from build123d import *

# Parameters (mm, degrees)
F0_W     = 66.675
F0_H     = 101.6
F1_DEPTH = 0.79375


with BuildPart() as f1:
    # F0 (on Front) → F1 (new body, symmetric)
    with BuildSketch(Plane.XZ):
        with BuildLine():
            Line((117.475, 114.3), (-117.475, 114.3))
            ThreePointArc((-117.475, 114.3), (-126.455256, 110.580256), (-130.175, 101.6))
            Line((-130.175, 101.6), (-130.175, -101.6))
            ThreePointArc((-130.175, -101.6), (-126.455256, -110.580256), (-117.475, -114.3))
            Line((-117.475, -114.3), (117.475, -114.3))
            Line((117.475, -114.3), (130.175, -114.3))
            Line((130.175, -114.3), (130.175, -101.6))
            Line((130.175, -101.6), (130.175, 101.6))
            Line((130.175, 101.6), (130.175, 114.3))
            Line((130.175, 114.3), (117.475, 114.3))
        make_face()
        with Locations((52.3875, -44.45)):
            Rectangle(F0_W, F0_H, mode=Mode.SUBTRACT)
    extrude(amount=F1_DEPTH, both=True)


solid = f1.part
For this review, take the finished solid that the model builds, in its own axes (mm). Round coordinates to 2 decimals unless told otherwise and drop trailing zeros. Write each loop counter-clockwise with the first axis right and the second up, starting at its lowest first coordinate (ties: lowest second). Pieces come first, ordered by that corner, then holes. Notation, with made-up numbers: (-23, 22) - (18, 22) arc R23 ccw to (18, 35) - close; hole circle Ø2 at (-3, -3.5). An arc over 180 degrees is marked (long way). Use a Markdown table: item, result.
Q1. Wall thickness on line 1 along X through (y, z) = (0.6, -87.5) (3 decimals); line 2 along Z through (x, y) = (84, 0): over which ranges is each line inside the solid? List them lowest first.
Derived:
| item | result |
|---|---|
| line 1 | x = -130.175 to 19.05, 85.725 to 130.175 |
| line 2 | z = -114.3 to -95.25, 6.35 to 114.3 |
Q2. We need section A-A (z = -39). Give the boundary of the cut face in (x, y) (3 decimals).
Derived:
| item | result |
|---|---|
| outline | (-130.175, -0.794) - (19.05, -0.794) - (19.05, 0.794) - (-130.175, 0.794) - close; (85.725, -0.794) - (130.175, -0.794) - (130.175, 0.794) - (85.725, 0.794) - close |
Q3. We need section C-C (y = -0.15). Give the boundary of the cut face in (x, z) (3 decimals), plus the area to 3 significant figures.
Derived:
| item | result |
|---|---|
| outline | (-130.175, -101.6) arc R12.7 ccw to (-117.475, -114.3) - (130.175, -114.3) - (130.175, 114.3) - (-117.475, 114.3) arc R12.7 ccw to (-130.175, 101.6) - close; hole (19.05, -95.25) - (85.725, -95.25) - (85.725, 6.35) - (19.05, 6.35) - close |
| area | 52,700 mm2 |
Q4. We need section B-B (x = 27). Give the boundary of the cut face in (y, z), plus the area to 3 significant figures.
Derived:
| item | result |
|---|---|
| outline | (-0.79, -114.3) - (0.79, -114.3) - (0.79, -95.25) - (-0.79, -95.25) - close; (-0.79, 6.35) - (0.79, 6.35) - (0.79, 114.3) - (-0.79, 114.3) - close |
| area | 202 mm2 |
